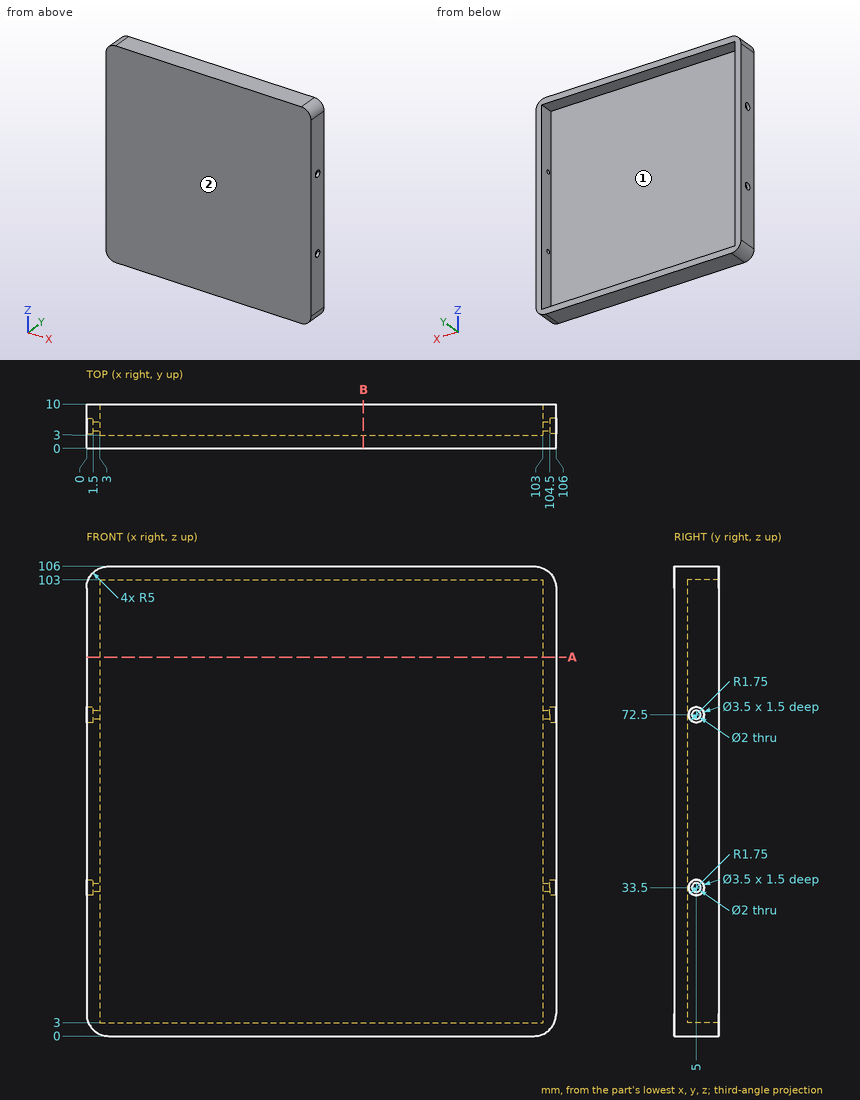
Geometry: see drawing. Coordinates: mm, zero at the bounding-box minimum. Coordinates: 2 decimals unless noted, no trailing zeros. Order: outer loops, then holes, each group sorted by start corner. A loop starts at its lowest first (then second) coordinate and runs counter-clockwise, first axis right, second up. Notation, with made-up numbers: M -16.75,61.5 L 34.25,61.5 A11 cw 34.25,81.5 Z; hole C -32.5,-25.5 d4. An arc over 180 degrees is marked long. Answer in a Markdown table with one row per item. Add a question column.
Q1. Line query: L1, parallel to Z at x = 80, y = 5.75; L2, parallel to Y at x = 103.3, z = 72.5. Output: solid intervals per line, ascending.
Q2. Section query A-A on z = 85.5. Return the cut outline in (x, y), and give its area (3 significant figures).
Q3. Section query B-B on x = 62.5. Return the cut outline in (y, z).
Q4. Mould query, pull axis X, two halves, no side actions, for the marked faces 1 and 2. Classes: released by +X, released by -X, zero draft, split by the parting line, or undercut.
Q5. Contact query for flat-ended pins moving along their axis: P1, Ø8, axis at x = 64.5, z = 82, coming from the -Y side; P2, Ø2, axis at x = 51, z = 56, coming from the +Y side; P3, Ø2.5, axis at y = 5, z = 72.5, coming from the +X side; P4, Ø3, axis at y = 5, z = 72.5, coming from the -X side. Output: stop coordinate, or through.
Completed:
| question | item | result |
|---|---|---|
| 1 | L1 | z = 0 to 3, 103 to 106 |
| 1 | L2 | y = 0 to 4, 6 to 10 |
| 2 | outline | M 0,0 L 106,0 L 106,10 L 103,10 L 103,3 L 3,3 L 3,10 L 0,10 Z |
| 2 | area | 360 mm2 |
| 3 | outline | M 0,0 L 10,0 L 10,3 L 3,3 L 3,103 L 10,103 L 10,106 L 0,106 Z |
| 4 | face 1 | undercut |
| 4 | face 2 | zero draft |
| 5 | P1 | stops at y = 0 |
| 5 | P2 | stops at y = 3 |
| 5 | P3 | stops at x = 104.5 |
| 5 | P4 | stops at x = 1.5 |
